```python
from build123d import *

# Parameters (mm, degrees)
SKETCH1_R           = 31.0896
BOSS_EXTRUDE1_DEPTH = 34.925
BOSS_EXTRUDE2_START = -30.48
BOSS_EXTRUDE2_DEPTH = 30.48
BOSS_EXTRUDE3_DEPTH = 34.925
CUT_EXTRUDE1_REACH  = 122.634
SKETCH4_R           = 6.35
SKETCH4_R_2         = 1.778
SKETCH5_W           = 18.49932761
SKETCH5_H           = 18.49932761
CUT_EXTRUDE2_DEPTH  = 34.925
FILLET3_R           = 2.54
FILLET4_R           = 2.54
FILLET5_R           = 2.54
FILLET6_R           = 2.54
FILLET8_R           = 6.35
FILLET9_R           = 6.35
FILLET10_R          = 6.35
CUT_EXTRUDE3_START  = -19.05
CUT_EXTRUDE3_DEPTH  = 19.05
CUT_EXTRUDE4_DEPTH  = 11.43
CUT_EXTRUDE5_DEPTH  = 11.43


with BuildPart() as part:
    # Sketch1 → Boss-Extrude1 (new body)
    with BuildSketch(Plane(origin=(0, 0, 0), x_dir=(1, 0, 0), z_dir=(0, 1, 0))):
        with Locations(Location((0, 0, 0), (0, 0, 270))):
            Circle(SKETCH1_R)
    extrude(amount=BOSS_EXTRUDE1_DEPTH)

    # Sketch2 → Boss-Extrude2 (add)
    with BuildSketch(Plane(origin=(0, 34.925, 0), x_dir=(1, 0, 0), z_dir=(0, 1, 0)).offset(BOSS_EXTRUDE2_START)):
        with BuildLine():
            Line((46.542690567, -48.26), (17.1704, -48.26))
            ThreePointArc((17.1704, -48.26), (-16.95457326, -34.12497326), (-31.0896, 0))
            ThreePointArc((-31.0896, 0), (1.271062728, -31.063606161), (30.985668109, 2.54))
            Line((30.985668109, 2.54), (46.542690567, 2.54))
            Line((46.542690567, 2.54), (46.542690567, -48.26))
        make_face()
    extrude(amount=BOSS_EXTRUDE2_DEPTH)

    # Sketch3 → Boss-Extrude3 (add)
    with BuildSketch(Plane(origin=(0, 34.925, 0), x_dir=(1, 0, 0), z_dir=(0, 1, 0))):
        Polygon((46.542690567, -0.333607673), (46.542690567, -48.26), (103.692690567, -48.26), (103.692690567, -41.91), (52.892690567, -41.91), (52.892690567, -3.81), (103.692690567, -3.81), (103.692690567, 2.54), (46.542690567, 2.54), align=None)
    extrude(amount=-BOSS_EXTRUDE3_DEPTH)

    # Cut-Extrude1: up to this face of the body (flat: up to its plane)
    cut_extrude1_end = Plane(part.part.faces().sort_by_distance((61.721911557, 18.150695346, 48.26))[0])
    # Sketch4 → Cut-Extrude1 (cut, up to the picked face)
    with BuildSketch(Plane(origin=(0, 0, -2.54), x_dir=(-1, 0, 0), z_dir=(0, 0, -1)), mode=Mode.PRIVATE) as cut_extrude1_sk1:
        with Locations((-92.262690567, 17.4625)):
            Circle(SKETCH4_R)
    cut_extrude1_tool1 = split(extrude(cut_extrude1_sk1.sketch, amount=-CUT_EXTRUDE1_REACH, mode=Mode.PRIVATE), bisect_by=cut_extrude1_end, keep=Keep.BOTH, mode=Mode.PRIVATE)
    # Sketch4 → Cut-Extrude1 (cut, up to the picked face)
    with BuildSketch(Plane(origin=(0, 0, -2.54), x_dir=(-1, 0, 0), z_dir=(0, 0, -1)), mode=Mode.PRIVATE) as cut_extrude1_sk2:
        with Locations((-85.347893353, 10.547702787)):
            Circle(SKETCH4_R_2)
    cut_extrude1_tool2 = split(extrude(cut_extrude1_sk2.sketch, amount=-CUT_EXTRUDE1_REACH, mode=Mode.PRIVATE), bisect_by=cut_extrude1_end, keep=Keep.BOTH, mode=Mode.PRIVATE)
    # Sketch4 → Cut-Extrude1 (cut, up to the picked face)
    with BuildSketch(Plane(origin=(0, 0, -2.54), x_dir=(-1, 0, 0), z_dir=(0, 0, -1)), mode=Mode.PRIVATE) as cut_extrude1_sk3:
        with Locations((-99.17748778, 24.377297213)):
            Circle(SKETCH4_R_2)
    cut_extrude1_tool3 = split(extrude(cut_extrude1_sk3.sketch, amount=-CUT_EXTRUDE1_REACH, mode=Mode.PRIVATE), bisect_by=cut_extrude1_end, keep=Keep.BOTH, mode=Mode.PRIVATE)
    # Sketch4 → Cut-Extrude1 (cut, up to the picked face)
    with BuildSketch(Plane(origin=(0, 0, -2.54), x_dir=(-1, 0, 0), z_dir=(0, 0, -1)), mode=Mode.PRIVATE) as cut_extrude1_sk4:
        with Locations((-99.17748778, 10.547702787)):
            Circle(SKETCH4_R_2)
    cut_extrude1_tool4 = split(extrude(cut_extrude1_sk4.sketch, amount=-CUT_EXTRUDE1_REACH, mode=Mode.PRIVATE), bisect_by=cut_extrude1_end, keep=Keep.BOTH, mode=Mode.PRIVATE)
    # Sketch4 → Cut-Extrude1 (cut, up to the picked face)
    with BuildSketch(Plane(origin=(0, 0, -2.54), x_dir=(-1, 0, 0), z_dir=(0, 0, -1)), mode=Mode.PRIVATE) as cut_extrude1_sk5:
        with Locations((-85.347893353, 24.377297213)):
            Circle(SKETCH4_R_2)
    cut_extrude1_tool5 = split(extrude(cut_extrude1_sk5.sketch, amount=-CUT_EXTRUDE1_REACH, mode=Mode.PRIVATE), bisect_by=cut_extrude1_end, keep=Keep.BOTH, mode=Mode.PRIVATE)
    add(cut_extrude1_tool1.solids().sort_by(Axis((92.262691, 17.4625, -2.54), (0, 0, 1)))[0], mode=Mode.SUBTRACT)
    add(cut_extrude1_tool2.solids().sort_by(Axis((85.347893, 10.547703, -2.54), (0, 0, 1)))[0], mode=Mode.SUBTRACT)
    add(cut_extrude1_tool3.solids().sort_by(Axis((99.177488, 24.377297, -2.54), (0, 0, 1)))[0], mode=Mode.SUBTRACT)
    add(cut_extrude1_tool4.solids().sort_by(Axis((99.177488, 10.547703, -2.54), (0, 0, 1)))[0], mode=Mode.SUBTRACT)
    add(cut_extrude1_tool5.solids().sort_by(Axis((85.347893, 24.377297, -2.54), (0, 0, 1)))[0], mode=Mode.SUBTRACT)

    # Sketch5 → Cut-Extrude2 (cut)
    with BuildSketch(Plane(origin=(0, 34.925, 0), x_dir=(1, 0, 0), z_dir=(0, 1, 0))):
        Rectangle(SKETCH5_W, SKETCH5_H)
    extrude(amount=-CUT_EXTRUDE2_DEPTH, mode=Mode.SUBTRACT)

    # Fillet3
    fillet3_edges = [part.edges().sort_by_distance(p)[0] for p in [
        (-9.249663805, 17.4625, 9.249663805),
    ]]
    fillet(fillet3_edges, radius=FILLET3_R)

    # Fillet4
    fillet4_edges = [part.edges().sort_by_distance(p)[0] for p in [
        (-9.249663805, 17.4625, -9.249663805),
    ]]
    fillet(fillet4_edges, radius=FILLET4_R)

    # Fillet5
    fillet5_edges = [part.edges().sort_by_distance(p)[0] for p in [
        (9.249663805, 17.4625, -9.249663805),
    ]]
    fillet(fillet5_edges, radius=FILLET5_R)

    # Fillet6
    fillet6_edges = [part.edges().sort_by_distance(p)[0] for p in [
        (9.249663805, 17.4625, 9.249663805),
    ]]
    fillet(fillet6_edges, radius=FILLET6_R)

    # Fillet8
    fillet8_edges = [part.edges().sort_by_distance(p)[0] for p in [
        (30.985668109, 19.685, -2.54),
    ]]
    fillet(fillet8_edges, radius=FILLET8_R)

    # Fillet9
    fillet9_edges = [part.edges().sort_by_distance(p)[0] for p in [
        (52.892690567, 17.4625, 41.91),
    ]]
    fillet(fillet9_edges, radius=FILLET9_R)

    # Fillet10
    fillet10_edges = [part.edges().sort_by_distance(p)[0] for p in [
        (52.892690567, 17.4625, 3.81),
    ]]
    fillet(fillet10_edges, radius=FILLET10_R)

    # Sketch6 → Cut-Extrude3 (cut)
    with BuildSketch(Plane(origin=(0, 34.925, 0), x_dir=(1, 0, 0), z_dir=(0, 1, 0)).offset(CUT_EXTRUDE3_START)):
        with BuildLine():
            ThreePointArc((49.910134647, -8.255), (49.765923709, -9.202652137), (49.717690567, -10.16))
            Line((49.717690567, -10.16), (49.717690567, -35.56))
            ThreePointArc((49.717690567, -35.56), (49.765923709, -36.517347863), (49.910134647, -37.465))
            ThreePointArc((49.910134647, -37.465), (48.60711955, -42.751092628), (43.6884307, -45.085))
            Line((43.6884307, -45.085), (17.1704, -45.085))
            ThreePointArc((17.1704, -45.085), (-14.70950923, -31.87990923), (-27.9146, 0))
            ThreePointArc((-27.9146, 0), (-3.338101965, 27.714291772), (27.116241813, 6.628297151))
            ThreePointArc((27.116241813, 6.628297151), (30.48737672, 1.397725825), (36.368826599, -0.635))
            Line((36.368826599, -0.635), (43.6884307, -0.635))
            ThreePointArc((43.6884307, -0.635), (48.60711955, -2.968907372), (49.910134647, -8.255))
        make_face()
        with BuildLine():
            ThreePointArc((6.709663805, 9.249663805), (8.505715029, 8.505715029), (9.249663805, 6.709663805))
            Line((9.249663805, 6.709663805), (9.249663805, -6.709663805))
            ThreePointArc((9.249663805, -6.709663805), (8.505715029, -8.505715029), (6.709663805, -9.249663805))
            Line((6.709663805, -9.249663805), (-6.709663805, -9.249663805))
            ThreePointArc((-6.709663805, -9.249663805), (-8.505715029, -8.505715029), (-9.249663805, -6.709663805))
            Line((-9.249663805, -6.709663805), (-9.249663805, 6.709663805))
            ThreePointArc((-9.249663805, 6.709663805), (-8.505715029, 8.505715029), (-6.709663805, 9.249663805))
            Line((-6.709663805, 9.249663805), (6.709663805, 9.249663805))
        make_face(mode=Mode.SUBTRACT)
    extrude(amount=CUT_EXTRUDE3_DEPTH, mode=Mode.SUBTRACT)

    # Sketch8 → Cut-Extrude4 (cut)
    with BuildSketch(Plane(origin=(0, 15.875, 0), x_dir=(1, 0, 0), z_dir=(0, 1, 0))):
        with BuildLine():
            Line((22.412690567, -2.54), (41.462690567, -2.54))
            ThreePointArc((41.462690567, -2.54), (45.952818627, -4.399871939), (47.812690567, -8.89))
            Line((47.812690567, -8.89), (47.812690567, -36.83))
            ThreePointArc((47.812690567, -36.83), (45.952818627, -41.320128061), (41.462690567, -43.18))
            Line((41.462690567, -43.18), (22.412690567, -43.18))
            ThreePointArc((22.412690567, -43.18), (17.922562506, -41.320128061), (16.062690567, -36.83))
            Line((16.062690567, -36.83), (16.062690567, -8.89))
            ThreePointArc((16.062690567, -8.89), (17.922562506, -4.399871939), (22.412690567, -2.54))
        make_face()
    extrude(amount=-CUT_EXTRUDE4_DEPTH, mode=Mode.SUBTRACT)

    # Sketch9 → Cut-Extrude5 (cut)
    with BuildSketch(Plane(origin=(0, 15.875, 0), x_dir=(1, 0, 0), z_dir=(0, 1, 0))):
        with BuildLine():
            Line((-9.337309433, 20.679663805), (-9.337309433, 16.320204994))
            ThreePointArc((-9.337309433, 16.320204994), (-7.477437494, 11.830076933), (-2.987309433, 9.970204994))
            Line((-2.987309433, 9.970204994), (3.362690567, 9.970204994))
            ThreePointArc((3.362690567, 9.970204994), (7.852818627, 11.830076933), (9.712690567, 16.320204994))
            Line((9.712690567, 16.320204994), (9.712690567, 20.679663805))
            ThreePointArc((9.712690567, 20.679663805), (7.852818627, 25.169791865), (3.362690567, 27.029663805))
            Line((3.362690567, 27.029663805), (-2.987309433, 27.029663805))
            ThreePointArc((-2.987309433, 27.029663805), (-7.477437494, 25.169791865), (-9.337309433, 20.679663805))
        make_face()
    extrude(amount=-CUT_EXTRUDE5_DEPTH, mode=Mode.SUBTRACT)


solid = part.part
```
The model under review builds one solid part; all positions refer to its coordinate system, in mm. A direction names the side the tool comes from. Round coordinates to 2 decimals unless told otherwise and drop trailing zeros. Loops run counter-clockwise (first coordinate to the right, second up) from the corner with the lowest first, then second, coordinate; pieces in that order, holes last. Notation, with made-up numbers: M -38,66 L -15,66 A19 cw -15,102 Z; hole C 36.25,85.5 d6. An arc over 180 degrees is marked long. Put each result on its own line as item: value.
Q1. Consider section A-A, the plane x = 73. Give the boundary of the cut face in (y, z) (3 decimals), then the cut area to 3 significant figures.
Result set:
outline: M 0,-2.54 L 34.925,-2.54 L 34.925,3.81 L 0,3.81 Z; M 0,41.91 L 34.925,41.91 L 34.925,48.26 L 0,48.26 Z
area: 444 mm²
Q2. Machinability: for faces 5 (the cylindrical face through (54.802, 17.218, 40.099)), 6 (the cylindrical face through (8.525, 7.826, 8.486)), 7 (the flat face through (46.543, 2, 23)), 8 (the cylindrical face through (48.56, 25.27, 2.91)), which of the approach directions +Z, -Z, +X, -X, +Y, -Y give a long, thin tool a straight path to every point of the face, cutting with its end or side? Answer none if there is none.
Result set:
face 5: +X, +Y, -Y
face 6: +Y, -Y
face 7: +Z, -Z, -Y
face 8: +Y
Q3. For pin 1 (3 mm diameter, centred on x = 99.18, y = 24.38, fed in from +Z); pin 2 (17.5 mm diameter, centred on x = 87, y = 14, fed in from -Z); pin 3 (5 mm diameter, centred on x = -1, y = 11.5, fed in from +Z) (3 decimals); pin 4 (3.5 mm diameter, centred on y = 9.5, z = -19, fed in from -X), all flat-tipped, find the tip position at first contact; note any pin that passes through.
Result set:
pin 1: passes through
pin 2: stops at z = -2.54
pin 3: stops at z = 45.645
pin 4: stops at x = -25.87
Q4. To check wall thickness, follow L1, parallel to Z at x = 77.5, y = 26; L2, parallel to X at y = 16, z = -1.5; L3, parallel to X at y = 10, z = 2.5. State the ranges of each line that lie inside material, in increasing order.
Result set:
L1: z = -2.54 to 3.81, 41.91 to 48.26
L2: x = -31.05 to -27.87, 30.36 to 86.08, 98.44 to 103.69
L3: x = -31.02 to -9.25, 9.25 to 83.66, 87.04 to 97.49, 100.87 to 103.69
Q5. Consider section B-B, the plane z = 16.5. Give the boundary of the cut face in (x, y) (3 decimals).
Result set:
outline: M -28.181,4.445 L -26.35,4.445 L -26.35,0 L 26.35,0 L 26.35,4.445 L 16.063,4.445 L 16.063,15.875 L -24.787,15.875 L -24.787,34.925 L -28.181,34.925 Z; M 46.543,0 L 52.893,0 L 52.893,34.925 L 49.718,34.925 L 49.718,15.875 L 47.813,15.875 L 47.813,4.445 L 46.543,4.445 Z
Q6. Mouldability with a two-part tool opening along X and no side actions: class faces 1 (the flat face through (0, 8, -9.25)), 2 (the flat face through (60, 18, 48.26)), 3 (the flat face through (0, 10, -9.97)), 4 (the cylindrical face through (32.401, 19.898, -3.932)) as released by +X, released by -X, zero draft, split by the parting line, or undercut.
Result set:
face 1: undercut
face 2: zero draft
face 3: undercut
face 4: released by +X
Q7. Consider section C-C, the plane x = -13. Give the boundary of the cut face in (y, z) (3 decimals), then the cut area to 3 significant figures.
Result set:
outline: M 0,-28.241 L 34.925,-28.241 L 34.925,-24.703 L 15.875,-24.703 L 15.875,33.502 L 34.925,33.502 L 34.925,37.667 L 4.445,37.667 L 4.445,28.241 L 0,28.241 Z
area: 1,150 mm²
